Geometry: final body of the model. Coordinates: model frame, mm. A direction names the side the tool comes from. Give positions to 0.01 mm unless a question says otherwise; leave off trailing zeros. Write each loop counter-clockwise with the first axis right and the second up, starting at its lowest first coordinate (ties: lowest second). Pieces come first, ordered by that corner, then holes. Notation, with made-up numbers: M -1,2.5 L 46,2.5 A31 cw 46,28.5 Z; hole C 39,5 d10. An arc over 180 degrees is marked long. Use a Markdown table: item, result. Add a question column.
1) Section A-A on x = -7. Return the cut outline in (y, z), then the cut area to 3 significant figures.
2) Draft query along X for faces 3 (the flat face through (-7, 88.147, 5)), 4 (the cylindrical face through (-7.145, 26.444, 4.93)), 5 (the flat face through (0, 41.8, 13.9)). Return one class per face: +X half, -X half, draft (parallel to the pull), parting line (faces both ways), or undercut.
3) Line query: line 1 (Y direction, x = -7, z = 4.25); line 2 (Z direction, x = -1.5, y = 51); line 3 (Y direction, x = -5.5, z = 5). Output: solid intervals per line, ascending.
4) Section C-C on y = 55. Return the cut outline in (x, z), then the cut area to 3 significant figures.
5) Pin query (flat end, axial travel): pin 1 (3.5 mm diameter, centred on x = -4.5, y = 80.5, fed in from +Z); pin 2 (1 mm diameter, centred on x = -12, y = 65.5, fed in from -Z); pin 3 (6 mm diameter, centred on x = -7.5, z = 27, fed in from +Y); pin 4 (2 mm diameter, centred on x = -11.5, z = 25.5, fed in from -Y). Return the tip coordinate at first contact, or that it passes through.
6) Section D-D on z = 13.5. Return the cut outline in (x, y), then the cut area to 3 significant figures.
7) Set-up query: faces 1 (the flat face through (-7, 50, 35)), 2 (the cylindrical face through (-7.24, 28.64, 16.33)). Return all of +Z, -Z, +X, -X, +Y, -Y with unobstructed straight access to the full face (end or side cutting, diameter ignored); none if empty.
8) Section B-B on z = 18. Return the cut outline in (x, y), then the cut area to 3 significant figures.
Autodesk Inventor part; units mm, degrees
ref_plane "YZ Plane" through (0, 0, 0) normal (1, 0, 0) x (0, 1, 0)
ref_plane "XZ Plane" through (0, 0, 0) normal (0, 1, 0) x (-1, 0, 0)
ref_plane "XY Plane" through (0, 0, 0) normal (0, 0, 1) x (1, 0, 0)
sketch "Sketch1" plane through (0, 0, 0) normal (0, 0, 1) x (1, 0, 0)
  point P0 (0, 0)
sketch "Sketch2" plane through (0, 0, 0) normal (1, 0, 0) x (0, 1, 0)
  line L0 (13.1468, 0) -> (76.0129, 0)
  line L1 (13.1468, 0) -> (88.1468, 0)
  circle A0 centre (50.6468, 19) radius 10
  line L2 (13.1468, 35) -> (88.1468, 35)
  line L3 (13.1468, 0) -> (13.1468, 35)
  line L4 (88.1468, 0) -> (88.1468, 35)
  point P0 (0, 0)
  point P1 (90.0129, 0)
  dimension "d0" = 75
  dimension "d1" = 20
  dimension "d3" = 16
  dimension "d5" = 35
  dimension "d8" = 37.5
extrude "Extrusion1" add sketch "Sketch2" against normal blind 14
sketch "Sketch3" plane through (0, 13.1468, 35) normal (0, 0, 1) x (1, 0, 0)
  line L0 (0, 75) -> (0, 0)
  line L1 (0, 75) -> (-14, 75)
  line L2 (-14, 0) -> (-14, 75)
  line L3 (0, 0) -> (-14, 0)
  line L4 (0, 75) -> (0, 0)
  line L5 (0, 37.5) -> (-14, 37.5)
  point P0 (0, -13.1468)
  point P1 (-7, 10)
  point P2 (-7, 65)
  dimension "d12" = 7
  dimension "d13" = 14
  dimension "d14" = 10
hole "Hole1" at (-7, 23.1468, 35) at (-7, 78.1468, 35) direction (0, 0, -1) diameter 6.6 end through all counterbore diameter 11 counterbore depth 25
chamfer "Chamfer1" distance 24 angle 45 2 edges at (-7, 13.1468, 35) (-7, 88.1468, 35)
equation "\"d8\" = 0.5 * d0"
properties part number "Glidelejrehus" material "Steel, Galvanized"
Found:
| question | item | result |
|---|---|---|
| 1 | outline | M 13.15,0 L 19.85,0 L 19.85,10 L 17.65,10 L 17.65,15.5 L 13.15,11 Z; M 26.45,0 L 74.85,0 L 74.85,10 L 72.65,10 L 72.65,26.5 L 64.15,35 L 37.15,35 L 28.65,26.5 L 28.65,10 L 26.45,10 Z; M 81.45,0 L 88.15,0 L 88.15,11 L 83.65,15.5 L 83.65,10 L 81.45,10 Z; hole C 50.65,19 d20 |
| 1 | area | 1,360 mm² |
| 2 | face 3 | draft |
| 2 | face 4 | undercut |
| 2 | face 5 | +X half |
| 3 | line 1 | 13.15 to 19.85, 26.45 to 74.85, 81.45 to 88.15 |
| 3 | line 2 | 0 to 9.01, 28.99 to 35 |
| 3 | line 3 | 13.15 to 20.21, 26.09 to 75.21, 81.09 to 88.15 |
| 4 | outline | M -14,0 L 0,0 L 0,10 L -14,10 Z; M -14,28 L 0,28 L 0,35 L -14,35 Z |
| 4 | area | 238 mm² |
| 5 | pin 1 | z = 10 |
| 5 | pin 2 | z = 0 |
| 5 | pin 3 | y = 73.61 |
| 5 | pin 4 | y = 26.65 |
| 6 | outline | M -14,15.65 L 0,15.65 L 0,42.3 L -14,42.3 Z; M -14,59 L 0,59 L 0,85.65 L -14,85.65 Z; hole C -7,23.15 d11; hole C -7,78.15 d11 |
| 6 | area | 556 mm² |
| 7 | face 1 | +Z, +X, -X, +Y, -Y |
| 7 | face 2 | +Z |
| 8 | outline | M -14,20.15 L -11.61,20.15 A5.5 cw long -2.39,20.15 L 0,20.15 L 0,40.7 L -14,40.7 Z; M -14,60.6 L 0,60.6 L 0,81.15 L -2.39,81.15 A5.5 cw long -11.61,81.15 L -14,81.15 Z |
| 8 | area | 418 mm² |
